Check sheet for the modelled part. Datum: model origin and axes. Units: mm. Face numbers are marked on the shaded views. Give positions to 0.01 mm unless a question says otherwise; leave off trailing zeros. Loops run counter-clockwise (first coordinate to the right, second up) from the corner with the lowest first, then second, coordinate; pieces in that order, holes last. Notation, with made-up numbers: M 69,-33 L 115,-33 A32 cw 115,-6 Z; hole C -0.75,-29 d5. An arc over 180 degrees is marked long. Write each question's results on one line, items separated by ' | '. Start each with the question number.
1. Go/stop test with flat-tipped pins: pin 1 (4 mm diameter, centred on x = 2.5, y = 25, fed in from -Z); pin 2 (1.5 mm diameter, centred on x = 3.5, y = 30, fed in from -Z); pin 3 (1.5 mm diameter, centred on x = -1.5, y = 25, fed in from +Z). Record where each tip stops, or that it passes through.
2. Sectioned sample at A-A on y = 3. Record the cut outline in (x, z), and give its area (3 significant figures).
3. Draft check along Y on the marked faces 1 and 2. Enter one of: pulls with the +Y half, pulls with the -Y half, needs draft (parallel to the pull), parting line crosses it, or undercut.
4. Material ranges on line 1 along X through (y, z) = (2, -3); line 2 along X through (y, z) = (32.5, 2); line 3 along Z through (x, y) = (-2, 23.5), recorded low to high.
5. Sectioned sample at B-B on y = 26.5. Record the cut outline in (x, z), and give its area (3 significant figures).
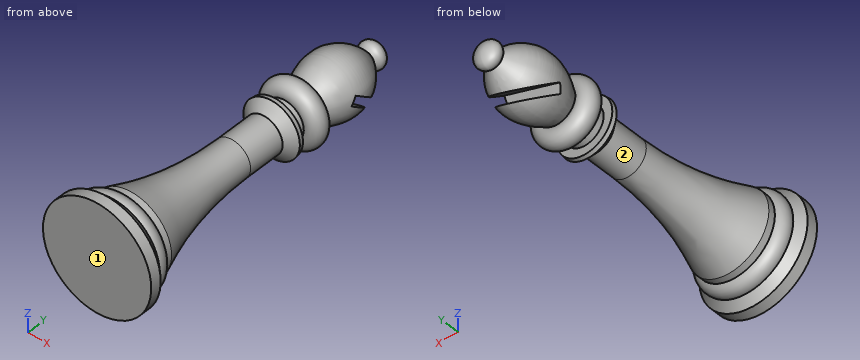
```python
from build123d import *
from OCP.BRepAlgoAPI import BRepAlgoAPI_Cut
from OCP.TopTools import TopTools_ListOfShape

# Parameters (mm, degrees)
CUT_EXTRUDE1_DEPTH      = 5.842
CUT_EXTRUDE1_DEPTH_BACK = 7.112


with BuildPart() as part:
    # Sketch1 → Revolve1 (revolve)
    with BuildSketch(Plane.XY, mode=Mode.PRIVATE) as revolve1_sk:
        with BuildLine():
            Line((0, 0), (6.35, 0))
            Line((6.35, 0), (6.35, 1.27))
            Line((6.35, 1.27), (5.451974388, 2.168025612))
            ThreePointArc((5.451974388, 2.168025612), (5.425268168, 3.139674583), (4.719324443, 3.807850011))
            Line((4.719324443, 3.807850011), (4.719324443, 4.618157389))
            add(Edge.make_bspline(
                [(4.719324443, 4.618157389), (2.191207341, 11.149425628), (2.162945217, 18.210926818)],
                knots=[0, 0, 0, 1, 1, 1], degree=2))
            Line((2.162945217, 18.210926818), (2.162945217, 22.528926818))
            Line((2.162945217, 22.528926818), (3.311767534, 23.530317493))
            Line((3.311767534, 23.530317493), (3.242795694, 24.033613514))
            Line((3.242795694, 24.033613514), (2.230740911, 24.033613514))
            Line((2.230740911, 24.033613514), (2.230740911, 25.303613514))
            ThreePointArc((2.230740911, 25.303613514), (3.755743451, 26.582465667), (2.162945217, 27.77581782))
            add(Edge.make_bspline(
                [(1.000273268, 36.229714038), (5.275414498, 32.931450332), (2.162945217, 27.77581782)],
                knots=[0, 0, 0, 1, 1, 1], degree=2))
            add(Edge.make_bspline(
                [(1.000273268, 36.229714038), (4.067898527, 38.111819372), (0, 38.111819372)],
                knots=[5.428894031, 5.428894031, 5.428894031, 7.853981634, 7.853981634, 7.853981634], degree=2, weights=[1, 0.35063824, 1]))
            Line((0, 38.111819372), (0, 38.1))
            Line((0, 38.1), (0, 0))
        make_face()
    revolve(revolve1_sk.sketch.rotate(Axis((0, 0, 0), (0, 1, 0)), 90), axis=Axis((0, 0, 0), (0, 1, 0)))


with BuildPart() as cut_extrude1_tool:
    # Sketch3 → Cut-Extrude1 (new, two sides: drawn at the far end of the back side and taken through both)
    with BuildSketch(Plane(origin=(-3.227609174, 24.033613514, -0.313469186), x_dir=(-0.29997267443447917, 0, 0.9539477944796696), z_dir=(-0.9539477944796697, 0, -0.29997267443447917)).offset(-CUT_EXTRUDE1_DEPTH_BACK)):
        with BuildLine():
            Line((-3.24447126, 10.581689828), (-0.778987351, 7.036762029))
            Line((-0.778987351, 7.036762029), (-1.61308801, 6.456648169))
            Line((-1.61308801, 6.456648169), (-3.788514988, 9.584525638))
            ThreePointArc((-3.788514988, 9.584525638), (-3.824633805, 10.251226491), (-3.24447126, 10.581689828))
        make_face()
    extrude(amount=CUT_EXTRUDE1_DEPTH + CUT_EXTRUDE1_DEPTH_BACK)


with BuildPart() as part_1:
    add(part.part)

    # Cut-Extrude1: cut by cut_extrude1_tool, with a tolerance
    cut_extrude1_stock = TopTools_ListOfShape()
    cut_extrude1_stock.Append(part_1.part.wrapped)
    cut_extrude1_tools = TopTools_ListOfShape()
    cut_extrude1_tools.Append(cut_extrude1_tool.part.wrapped)
    cut_extrude1_cut = BRepAlgoAPI_Cut()
    cut_extrude1_cut.SetArguments(cut_extrude1_stock)
    cut_extrude1_cut.SetTools(cut_extrude1_tools)
    cut_extrude1_cut.SetFuzzyValue(0.00001)
    cut_extrude1_cut.Build()
    add(Compound.cast(cut_extrude1_cut.Shape()).solids(), mode=Mode.REPLACE)


solid = part_1.part
```
Output values:
1) pin 1: z = -3.6 | pin 2: z = -1.68 | pin 3: z = 3.2
2) outline: C 0,0 d10.96 | area: 94.3 mm2
3) face 1: pulls with the -Y half | face 2: undercut
4) line 1: -4.75 to 4.75 | line 2: -2.78 to 2.78 | line 3: -2.6 to 2.6
5) outline: C 0,0 d7.51 | area: 44.3 mm2
